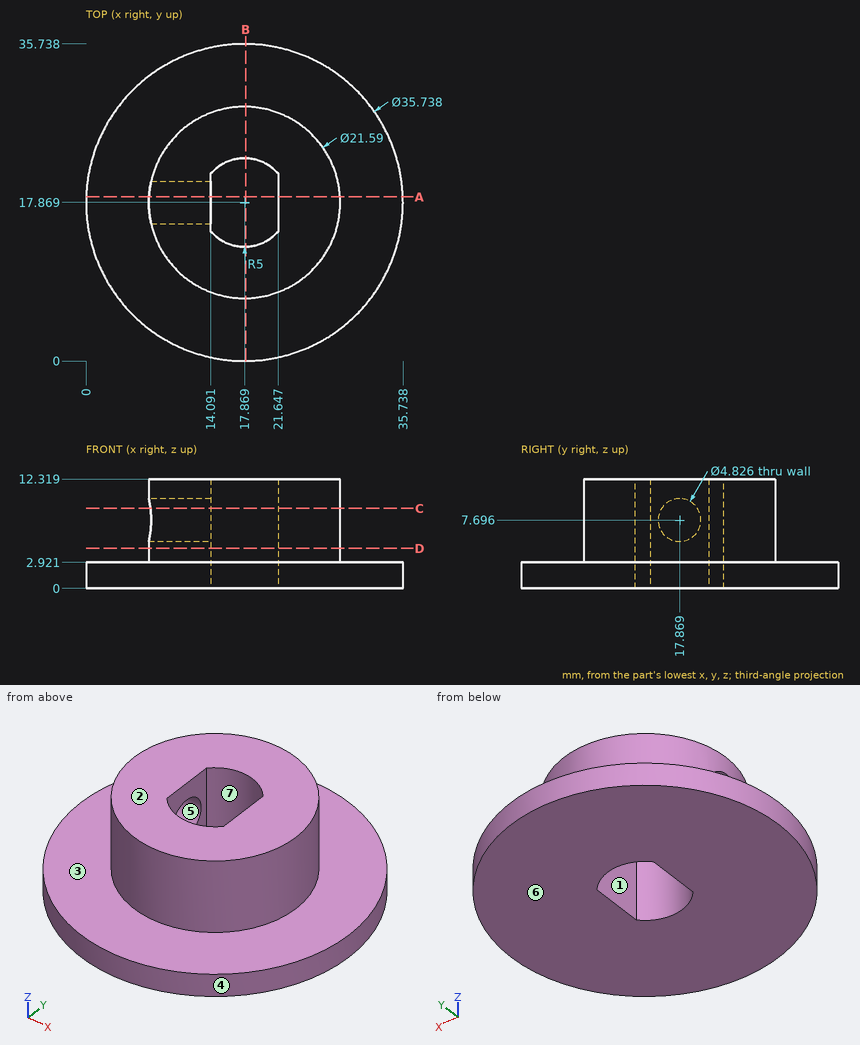
For this review, use the dimensioned drawing (mm, ordinates from the lowest corner) and the shaded views. A direction names the side the tool comes from. Round coordinates to 2 decimals unless told otherwise and drop trailing zeros. Write each loop counter-clockwise with the first axis right and the second up, starting at its lowest first coordinate (ties: lowest second). Pieces come first, ordered by that corner, then holes. Notation, with made-up numbers: M -13,48 L 8,48 A16 cw 8,63 Z; hole C -13.75,-24 d8. An arc over 180 degrees is marked long. Answer as CSV lines item,"result". Start each with the question number.
Q1. Wall thickness on line 1 along Z through (x, y) = (19, 4); line 2 along Y through (x, z) = (10, 8.5) (1 decimal); line 3 along X through (y, z) = (20, 6.25): over which ranges is each line inside the solid? List them lowest first.
Q2. Tool access review of the marked faces 1, 2 and 3: name each direction out of +Z, -Z, +X, -X, +Y, -Y from which nothing blocks a thin tool from reaching the whole face with its end or side.
Q3. The part is to be moulded in two halves that separate along Y. For the marked faces 4, 5, 6 and 7, say which applies: +Y half, -Y half, draft (parallel to the pull), parting line (faces both ways), or undercut.
Q4. Consider section D-D, the plane z = 4.5. Give the boundary of the cut face in (x, y) (1 decimal).
Q5. Clearance check with flat-ended pins moving along their axes: P1, Ø2, axis at y = 9.5, z = 7.5, coming from the +X side; P2, Ø12, axis at x = 14, y = 32, coming from the +Z side; P3, Ø5, axis at y = 16.5, z = 6, coming from the +X side; P4, Ø4, axis at y = 18, z = 8.5, coming from the -X side. State where each tip first meets the part, or that it passes through.
Q6. Consider section A-A, the plane y = 18.5. Give the boundary of the cut face in (x, z) (1 decimal).
Q7. Consider section B-B, the plane x = 18. Give the boundary of the cut face in (y, z) (1 decimal), then the cut area to 3 significant figures.
Q8. Consider section C-C, the plane z = 9. Give the boundary of the cut face in (x, y) (1 decimal).
Result set:
1,line 1,"z = 0 to 2.92"
1,line 2,"y = 10.5 to 15.6, 20.1 to 25.3"
1,line 3,"x = 7.29 to 14.09, 21.65 to 28.45"
2,face 1,"+Z, -Z"
2,face 2,"+Z, +X, -X, +Y, -Y"
2,face 3,"+Z"
3,face 4,"parting line"
3,face 5,"undercut"
3,face 6,"draft"
3,face 7,"undercut"
4,outline,"C 17.9,17.9 d21.6; hole M 14.1,14.6 A5 ccw 21.6,14.6 L 21.6,21.1 A5 ccw 14.1,21.1 Z"
5,P1,"stops at x = 25.76"
5,P2,"stops at z = 12.32"
5,P3,"stops at x = 28.66"
5,P4,"stops at x = 7.07"
6,outline,"M 0,0 L 14.1,0 L 14.1,5.4 L 7.1,5.4 L 7.1,2.9 L 0,2.9 Z; M 7.1,10 L 14.1,10 L 14.1,12.3 L 7.1,12.3 Z; M 21.6,0 L 35.7,0 L 35.7,2.9 L 28.6,2.9 L 28.6,12.3 L 21.6,12.3 Z"
7,outline,"M 0,0 L 12.9,0 L 12.9,12.3 L 7.1,12.3 L 7.1,2.9 L 0,2.9 Z; M 22.9,0 L 35.7,0 L 35.7,2.9 L 28.7,2.9 L 28.7,12.3 L 22.9,12.3 Z"
7,area,"184 mm²"
8,outline,"M 7.3,15.8 A10.8 ccw long 7.3,19.9 L 14.1,19.9 L 14.1,21.1 A5 cw 21.6,21.1 L 21.6,14.6 A5 cw 14.1,14.6 L 14.1,15.8 Z"
